```python
from build123d import *

# Parameters (mm, degrees)
SKETCH1_W          = 12.617819502
SKETCH1_H          = 2
SKETCH1_W_2        = 6.5532
SKETCH1_H_2        = 5.31
SKETCH2_R          = 1.0922
CUT_EXTRUDE1_DEPTH = 30.264206533
SKETCH3_W          = 45.123892984
SKETCH3_H          = 9
CUT_EXTRUDE2_DEPTH = 1
CHAMFER1_SIZE      = 0.5


with BuildPart() as part:
    # Sketch1 → Revolve1 (revolve)
    with BuildSketch(Plane(origin=(0, 0, 0), x_dir=(1, 0, 0), z_dir=(0, 1, 0))):
        with Locations((-13.308909751, 2.525473465)):
            Rectangle(SKETCH1_W, SKETCH1_H)
        Polygon((-11.938, 1.525473465), (-19.617819502, 1.525473465), (-19.617819502, -0.474526535), (-13.064619502, -0.474526535), (-11.938, -0.474526535), align=None)
        with Locations((-16.341219502, -3.129526535)):
            Rectangle(SKETCH1_W_2, SKETCH1_H_2)
    revolve(axis=Axis((0, 0, -25.411285606), (0, 0, 1)))

    # Sketch2 → Cut-Extrude1 (cut, through all)
    with BuildSketch(Plane(origin=(0, 0, -3.525473465), x_dir=(-1, 0, 0), z_dir=(0, 0, -1))):
        with Locations((16.57, 0)):
            Circle(SKETCH2_R)
        with Locations(Location((-16.57, 0, 0), (0, 0, 180))):
            Circle(SKETCH2_R)
    extrude(amount=-CUT_EXTRUDE1_DEPTH, mode=Mode.SUBTRACT)

    # Sketch3 → Cut-Extrude2 (cut)
    with BuildSketch(Plane(origin=(0, 0, -3.525473465), x_dir=(-1, 0, 0), z_dir=(0, 0, -1))):
        Rectangle(SKETCH3_W, SKETCH3_H)
    extrude(amount=-CUT_EXTRUDE2_DEPTH, mode=Mode.SUBTRACT)

    # Chamfer1
    chamfer1_edges = [part.edges().sort_by_distance(p)[0] for p in [
        (11.938, 0, 0.474526535),
    ]]
    chamfer(chamfer1_edges, length=CHAMFER1_SIZE)


solid = part.part
```
Verification items for the finished model (mm, model axes). A direction names the side the tool comes from. Round coordinates to 2 decimals unless told otherwise and drop trailing zeros. Order: outer loops, then holes, each group sorted by start corner. A loop starts at its lowest first (then second) coordinate and runs counter-clockwise, first axis right, second up. Notation, with made-up numbers: (8, -10) -> (28, -10) arc R10 ccw to (28, 2) -> close; hole circle Ø11 at (-16, -35.75). An arc over 180 degrees is marked (long way). Put each result on its own line as item: value. Start each with the question number.
(1) Depth check by flat-ended pin: pin 1 Ø2.5 at (x, y) = (-16.57, 0) entering from +Z; pin 2 Ø0.5 at (x, z) = (-10.5, -3) entering from +Y; pin 3 Ø7 at (x, y) = (1.5, 0.5) entering from +Z; pin 4 Ø5 at (y, z) = (8, 4) entering from -X. Enter the tip coordinate at first touch or a pass-through.
(2) Section check A-A (x = 0). Enter the section's corners in (y, z).
(3) Draft check along X on faces 1 (the face through (-5.1, 5.1, -1.525)), 2 (the face through (-18.712, -5.893, 1.195)), 3 (the face through (12, -4.5, -3)). Enter one of: +X half, -X half, draft (parallel to the pull), parting line (faces both ways), or undercut.
(4) Material ranges on line 1 along Y through (x, z) = (0, -2.1); line 2 along Y through (x, z) = (0, -0.5); line 3 along Z through (x, y) = (-9.5, -5), recorded low to high.
(5) Tool access check on faces 4 (the face through (-15.48, 0.05, 1.57)), 5 (the face through (-12, 0, -2.525)), 6 (the face through (2.588, 11.654, -0.786)). Record the directions out of +Z, -Z, +X, -X, +Y, -Y that give a thin tool (end or side, any length) a straight path to the whole face; none if there is none.
(6) Section check C-C (z = 2). Enter the section's corners in (x, y).
(7) Section check D-D (x = -16.57). Enter the section's corners in (y, z).
(8) Section check B-B (y = 0). Enter the section's corners in (x, z).
Completed:
1. pin 1: stops at z = 5.78
1. pin 2: stops at y = 16.73
1. pin 3: passes through
1. pin 4: stops at x = -18.83
2. outline: (-19.62, -3.53) -> (-7, -3.53) -> (-7, -1.53) -> (-11.94, -1.53) -> (-11.94, -0.03) -> (-12.44, 0.47) -> (-13.06, 0.47) -> (-13.06, 5.78) -> (-19.62, 5.78) -> close; (7, -3.53) -> (19.62, -3.53) -> (19.62, 5.78) -> (13.06, 5.78) -> (13.06, 0.47) -> (12.44, 0.47) -> (11.94, -0.03) -> (11.94, -1.53) -> (7, -1.53) -> close
3. face 1: undercut
3. face 2: parting line
3. face 3: draft
4. line 1: y = -19.62 to -7, 7 to 19.62
4. line 2: y = -19.62 to -11.94, 11.94 to 19.62
4. line 3: z = -3.53 to -1.53
5. face 4: +Z, -Z
5. face 5: -Z, +X, -X
5. face 6: +Z
6. outline: circle Ø39.24 at (0, 0); hole circle Ø2.18 at (-16.57, 0); hole circle Ø26.13 at (0, 0); hole circle Ø2.18 at (16.57, 0)
7. outline: (-10.5, -3.53) -> (-4.5, -3.53) -> (-4.5, -2.53) -> (-1.09, -2.53) -> (-1.09, 5.78) -> (-10.5, 5.78) -> close; (1.09, -2.53) -> (4.5, -2.53) -> (4.5, -3.53) -> (10.5, -3.53) -> (10.5, 5.78) -> (1.09, 5.78) -> close
8. outline: (-19.62, -2.53) -> (-17.66, -2.53) -> (-17.66, 5.78) -> (-19.62, 5.78) -> close; (-15.48, -2.53) -> (-7, -2.53) -> (-7, -1.53) -> (-11.94, -1.53) -> (-11.94, -0.03) -> (-12.44, 0.47) -> (-13.06, 0.47) -> (-13.06, 5.78) -> (-15.48, 5.78) -> close; (7, -2.53) -> (15.48, -2.53) -> (15.48, 5.78) -> (13.06, 5.78) -> (13.06, 0.47) -> (12.44, 0.47) -> (11.94, -0.03) -> (11.94, -1.53) -> (7, -1.53) -> close; (17.66, -2.53) -> (19.62, -2.53) -> (19.62, 5.78) -> (17.66, 5.78) -> close
